Geometry check sheet. Reference: the model listing, model coordinates, mm. A direction names the side the tool comes from. Coordinates: 2 decimals unless noted, no trailing zeros. Write each loop counter-clockwise with the first axis right and the second up, starting at its lowest first coordinate (ties: lowest second). Pieces come first, ordered by that corner, then holes. Notation, with made-up numbers: (0, 63) - (20, 63) arc R22 cw to (20, 70) - close; hole circle Ø11 at (25.25, 52.25). An arc over 180 degrees is marked (long way). Answer as a JSON object with one key per item and string values. Group by question number.
from build123d import *

# Parameters (mm, degrees)
SKETCH3_W                                       = 44.1
SKETCH3_H                                       = 30.1
BOSS_EXTRUDE1_DEPTH                             = 8
SKETCH4_W                                       = 44.1
SKETCH4_H                                       = 10
BOSS_EXTRUDE2_DEPTH                             = 25
CSK_FOR_M3_FLAT_HEAD_MACHINE_SCREW1_D           = 3.2
CSK_FOR_M3_FLAT_HEAD_MACHINE_SCREW1_CSINK_D     = 6.3
CSK_FOR_M3_FLAT_HEAD_MACHINE_SCREW1_CSINK_ANGLE = 90
SKETCH10_W                                      = 44.1
SKETCH10_H                                      = 8
BOSS_EXTRUDE3_DEPTH                             = 42.1
SKETCH11_R                                      = 11.25
CUT_EXTRUDE1_DEPTH                              = 42
M3_CLEARANCE_HOLE4_D                            = 3.2
BOSS_EXTRUDE4_DEPTH                             = 13
CHAMFER2_SIZE                                   = 2


with BuildPart() as part:
    # Sketch3 → Boss-Extrude1 (new body)
    with BuildSketch(Plane(origin=(0, 0, 0), x_dir=(1, 0, 0), z_dir=(0, 1, 0))):
        with Locations((0, -5)):
            Rectangle(SKETCH3_W, SKETCH3_H)
    extrude(amount=-BOSS_EXTRUDE1_DEPTH)

    # Sketch4 → Boss-Extrude2 (add)
    with BuildSketch(Plane.XZ.offset(8)):
        with Locations((0, 15.05)):
            Rectangle(SKETCH4_W, SKETCH4_H)
    extrude(amount=BOSS_EXTRUDE2_DEPTH)

    # CSK for M3 Flat Head Machine Screw1 (through all)
    with Locations(Plane(origin=(0, 0, 0), x_dir=(1, 0, 0), z_dir=(0, 1, 0))):
        with Locations((8, -7.5), (-8, -7.5), (8, 7.5), (-8, 7.5)):
            CounterSinkHole(CSK_FOR_M3_FLAT_HEAD_MACHINE_SCREW1_D / 2, CSK_FOR_M3_FLAT_HEAD_MACHINE_SCREW1_CSINK_D / 2, counter_sink_angle=CSK_FOR_M3_FLAT_HEAD_MACHINE_SCREW1_CSINK_ANGLE)

    # Sketch10 → Boss-Extrude3 (add)
    with BuildSketch(Plane(origin=(0, 0, 0), x_dir=(1, 0, 0), z_dir=(0, 1, 0))):
        with Locations((0, -16.05)):
            Rectangle(SKETCH10_W, SKETCH10_H)
    extrude(amount=BOSS_EXTRUDE3_DEPTH)

    # Sketch11 → Cut-Extrude1 (cut)
    with BuildSketch(Plane(origin=(0, 0, 12.05), x_dir=(-1, 0, 0), z_dir=(0, 0, -1))):
        with Locations((0, 21.05)):
            Circle(SKETCH11_R)
    extrude(amount=-CUT_EXTRUDE1_DEPTH, mode=Mode.SUBTRACT)

    # M3 Clearance Hole4 (through all)
    with Locations(Plane(origin=(0, 0, 12.05), x_dir=(-1, 0, 0), z_dir=(0, 0, -1))):
        with Locations((15.5, 5.55), (-15.5, 5.55), (15.5, 36.55), (-15.5, 36.55)):
            Hole(M3_CLEARANCE_HOLE4_D / 2)

    # Sketch14 → Boss-Extrude4 (add)
    with BuildSketch(Plane(origin=(22.05, 0, 0), x_dir=(0, 0, -1), z_dir=(1, 0, 0))):
        Polygon((10, 0), (-10, 0), (-12, 0), (-12, 42.1), (-20.05, 42.1), (-20.05, -6), (-12, -6), (-10, -6), (10, -6), align=None)
    extrude(amount=BOSS_EXTRUDE4_DEPTH)

    # Chamfer2
    chamfer2_edges = [part.edges().sort_by_distance(p)[0] for p in [
        (-22.05, -8, 0),
    ]]
    chamfer(chamfer2_edges, length=CHAMFER2_SIZE)


solid = part.part
(1) Section check D-D (x = 0). Record the cut outline in (y, z).
(2) Draft check along Z on faces 1 (the face through (-7.6, -1.303, -5.696)), 2 (the face through (1, -8, 0)), 3 (the face through (9, 30, 12.05)). Enter one of: +Z half, -Z half, draft (parallel to the pull), parting line (faces both ways), or undercut.
(3) Section check C-C (y = 36.55). Record the cut outline in (x, z), and give its area (3 significant figures).
(4) Section check B-B (z = 17). Record the cut outline in (x, y).
(5) Set-up check for faces 4 (the face through (8.35, -4.82, -5.94)), 5 (the face through (-21.06, -6.99, 0.14)), 6 (the face through (28, 21, 12)): record each of +Z, -Z, +X, -X, +Y, -Y from which the full face is reachable in a straight line by a thin tool's end or side.
(6) Section check A-A (y = 21.05). Record the cut outline in (x, z), and give its area (3 significant figures).
(7) Gauge pin test, flat ends, axial feed: pin 1 (21.5 mm diameter, centred on x = 9.5, y = -18.5, fed in from -Z); pin 2 (3 mm diameter, centred on x = 7.5, z = 9.5, fed in from +Y); pin 3 (12.5 mm diameter, centred on x = 2, y = 27, fed in from -Z); pin 4 (1.8 mm diameter, centred on x = 29.5, y = -4.5, fed in from -Z). Record the tip position at first contact, or that the pin passes through.
(8) Material ranges on L1, parallel to Y at x = 15.5, z = 15.25; L2, parallel to Z at x = 8, y = -4.25; L3, parallel to X at y = -3.25, z = -7.5, recorded low to high. Write a range as [from, to].
Conclusion:
{
 "1": {"outline": "(-33, 10.05) - (-8, 10.05) - (-8, -10.05) - (0, -10.05) - (0, 12.05) - (9.8, 12.05) - (9.8, 20.05) - (-33, 20.05) - close; (32.3, 12.05) - (42.1, 12.05) - (42.1, 20.05) - (32.3, 20.05) - close"},
 "2": {"face 1": "undercut", "face 2": "draft", "face 3": "-Z half"},
 "3": {"outline": "(-22.05, 12.05) - (-17.1, 12.05) - (-17.1, 20.05) - (-22.05, 20.05) - close; (-13.9, 12.05) - (13.9, 12.05) - (13.9, 20.05) - (-13.9, 20.05) - close; (17.1, 12.05) - (22.05, 12.05) - (22.05, 12) - (35.05, 12) - (35.05, 20.05) - (17.1, 20.05) - close", "area": "406 mm^2"},
 "4": {"outline": "(-22.05, -33) - (22.05, -33) - (22.05, -6) - (35.05, -6) - (35.05, 42.1) - (-22.05, 42.1) - close; hole circle Ø3.2 at (-15.5, 5.55); hole circle Ø3.2 at (-15.5, 36.55); hole circle Ø22.5 at (0, 21.05); hole circle Ø3.2 at (15.5, 5.55); hole circle Ø3.2 at (15.5, 36.55)"},
 "5": {"face 4": "+Y, -Y", "face 5": "-Z, -X, -Y", "face 6": "-Z, +X, -X, +Y"},
 "6": {"outline": "(-22.05, 12.05) - (-11.25, 12.05) - (-11.25, 20.05) - (-22.05, 20.05) - close; (11.25, 12.05) - (22.05, 12.05) - (22.05, 12) - (35.05, 12) - (35.05, 20.05) - (11.25, 20.05) - close", "area": "277 mm^2"},
 "7": {"pin 1": "stops at z = -10.05", "pin 2": "stops at y = 0", "pin 3": "stops at z = 12.05", "pin 4": "stops at z = -10"},
 "8": {"L1": "y = [-33, 3.95], [7.15, 34.95], [38.15, 42.1]", "L2": "z = [-10.05, -9.1], [-5.9, 5.9], [9.1, 20.05]", "L3": "x = [-22.05, -9.6], [-6.4, 6.4], [9.6, 35.05]"}
}
